Model file for the job. Use its own axes, mm. A direction names the side the tool comes from. Coordinates: 2 decimals unless noted, no trailing zeros. Write each loop counter-clockwise with the first axis right and the second up, starting at its lowest first coordinate (ties: lowest second). Pieces come first, ordered by that corner, then holes. Notation, with made-up numbers: (-27, 52) - (9, 52) arc R24 ccw to (9, 85) - close; hole circle Ø8 at (70, 21). An arc over 180 degrees is marked (long way). Put each result on its own line as item: value. Start each with the question number.
1. Saw through at B-B, the plane z = 0.75. Write the cut outline in (x, y), plus the area to 3 significant figures.
2. Which spindle directions (+Z, -Z, +X, -X, +Y, -Y) get a long thin tool onto all of the face, cutting with end or side? Do faces 4 (the face through (2, 2, -8)), 5 (the face through (-3, 0, 4)), 6 (the face through (1, -3, -2)). Say none if no direction does.
3. Saw through at A-A, the plane y = 0. Write the cut outline in (x, z), plus the area to 3 significant figures.
4. Drop flat-ended pins along their axis: P1, Ø2, axis at y = -3, z = 4.5, coming from the +X side; P2, Ø2, axis at y = -2, z = -6, coming from the -X side; P3, Ø3.5, axis at x = -0.5, y = 0, coming from the +Z side; P4, Ø3, axis at y = 0, z = -6, coming from the -X side. Give the stop position or say it passes through.
5. Drill centre lines: L1, parallel to X at y = 0, z = 1; L2, parallel to Y at x = 0, z = -2.25; L3, parallel to Z at x = -1.75, y = 2.5. Where is each one in solid material? Low to high. Write a range as from..to.
6. Pull direction Y, two halves, no side cores. Call faces 1 (the face through (1, -3, 2)), 2 (the face through (3, 0, -5)), 3 (the face through (2.44, 0.54, -1.1)): released by +Y, released by -Y, zero draft, split by the parting line, or undercut.
7. Saw through at D-D, the plane x = 2.75. Write the cut outline in (y, z), plus the area to 3 significant figures.
8. Saw through at C-C, the plane x = -0.5. Write the cut outline in (y, z), plus the area to 3 significant figures.
Autodesk Inventor part; units mm, degrees
ref_plane "YZ Plane" through (0, 0, 0) normal (1, 0, 0) x (0, 1, 0)
ref_plane "XZ Plane" through (0, 0, 0) normal (0, 1, 0) x (-1, 0, 0)
ref_plane "XY Plane" through (0, 0, 0) normal (0, 0, 1) x (1, 0, 0)
sketch "Sketch2" plane through (0, 0, 0) normal (0, 0, 1) x (1, 0, 0)
  line L0 (0, 4) -> (3.4641, 2)
  line L1 (3.4641, 2) -> (3.4641, -2)
  line L2 (3.4641, -2) -> (0, -4)
  line L3 (0, -4) -> (-3.4641, -2)
  line L4 (-3.4641, -2) -> (-3.4641, 2)
  line L5 (-3.4641, 2) -> (0, 4)
  point P0 (0, 0)
  point P1 (0, 0)
  point P2 (-3.4641, 0)
  dimension "d0" = 8
extrude "Extrusion1" add sketch "Sketch2" along normal mid plane 4
sketch "Sketch3" plane through (0, 0, 2) normal (0, 0, 1) x (1, 0, 0)
  circle A0 centre (0, 0) radius 3
  dimension "d3" = 6
extrude "Extrusion2" add sketch "Sketch3" along normal blind 4
sketch "Sketch4" plane through (0, 0, -2) normal (0, 0, -1) x (-1, 0, 0)
  circle A0 centre (0, 0) radius 3
  dimension "d6" = 6
extrude "Extrusion3" add sketch "Sketch4" along normal blind 6
sketch "Sketch5" plane through (0, 0, 6) normal (0, 0, 1) x (1, 0, 0)
  circle A0 centre (0, 0) radius 3
hole "Hole1" at (0, 0, 6) direction (0, 0, -1) diameter 5 depth 14
thread "Thread1"
properties part number "25.1"
Final values:
1. outline: (-3.46, -2) - (0, -4) - (3.46, -2) - (3.46, 2) - (0, 4) - (-3.46, 2) - close; hole circle Ø5 at (0, 0)
1. area: 21.9 mm²
2. face 4: -Z, +X, -X, +Y, -Y
2. face 5: +Z
2. face 6: -Z
3. outline: (-3.46, -2) - (-3, -2) - (-3, -8) - (-2.5, -8) - (-2.5, 6) - (-3, 6) - (-3, 2) - (-3.46, 2) - close; (2.5, -8) - (3, -8) - (3, -2) - (3.46, -2) - (3.46, 2) - (3, 2) - (3, 6) - (2.5, 6) - close
3. area: 17.7 mm²
4. P1: stops at x = 2.24
4. P2: stops at x = -2.83
4. P3: passes through
4. P4: stops at x = -3
5. L1: x = -3.46..-2.5, 2.5..3.46
5. L2: y = -3..-2.5, 2.5..3
5. L3: z = -2..2
6. face 1: zero draft
6. face 2: split by the parting line
6. face 3: undercut
7. outline: (-2.41, -2) - (-1.2, -2) - (-1.2, -8) - (1.2, -8) - (1.2, -2) - (2.41, -2) - (2.41, 2) - (1.2, 2) - (1.2, 6) - (-1.2, 6) - (-1.2, 2) - (-2.41, 2) - close
7. area: 43.3 mm²
8. outline: (-3.71, -2) - (-2.96, -2) - (-2.96, -8) - (-2.45, -8) - (-2.45, 6) - (-2.96, 6) - (-2.96, 2) - (-3.71, 2) - close; (2.45, -8) - (2.96, -8) - (2.96, -2) - (3.71, -2) - (3.71, 2) - (2.96, 2) - (2.96, 6) - (2.45, 6) - close
8. area: 20.3 mm²
